```python
from build123d import *

# Parameters (mm, degrees)
SKETCH1_R           = 12.7
BOSS_EXTRUDE1_DEPTH = 12.7
SKETCH2_R           = 1.6256
CUT_EXTRUDE1_DEPTH  = 9.525
SKETCH3_R           = 9.525
CUT_EXTRUDE2_DEPTH  = 2.54
BOSS_EXTRUDE2_START = -12.7
BOSS_EXTRUDE2_DEPTH = 12.7
SKETCH10_R          = 1.651
CUT_EXTRUDE4_DEPTH  = 12.7
SKETCH11_R          = 9.525
CUT_EXTRUDE5_DEPTH  = 5.18668
CUT_EXTRUDE6_DEPTH  = 12.7
FILLET1_R           = 3.175
SKETCH16_R          = 8.255
CUT_EXTRUDE8_DEPTH  = 3.175
SKETCH17_R          = 1.2192
CUT_EXTRUDE9_DEPTH  = 4.33832
SKETCH18_R          = 3.81
CUT_EXTRUDE10_DEPTH = 2.54


with BuildPart() as part:
    # Sketch1 → Boss-Extrude1 (new body)
    with BuildSketch(Plane(origin=(0, 0, 0), x_dir=(1, 0, 0), z_dir=(0, 1, 0))):
        with Locations(Location((0, 0, 0), (0, 0, 270))):
            Circle(SKETCH1_R)
    extrude(amount=BOSS_EXTRUDE1_DEPTH)

    # Sketch2 → Cut-Extrude1 (cut)
    with BuildSketch(Plane.XZ):
        with Locations(Location((0, 0, 0), (0, 0, 270))):
            Circle(SKETCH2_R)
    extrude(amount=-CUT_EXTRUDE1_DEPTH, mode=Mode.SUBTRACT)

    # Sketch3 → Cut-Extrude2 (cut)
    with BuildSketch(Plane.XZ):
        with Locations(Location((0, 0, 0), (0, 0, 270))):
            Circle(SKETCH3_R)
    extrude(amount=-CUT_EXTRUDE2_DEPTH, mode=Mode.SUBTRACT)

    # Sketch5 → #2-56 Tapped Hole1 (revolve, cut)
    with BuildSketch(Plane(origin=(0, 3.81, 0), x_dir=(0, 1, 0), z_dir=(1, 0, 0))):
        Polygon((0, 0), (0, 13.74216509), (0.889, 13.208), (0.889, 0), align=None)
    revolve(axis=Axis((0, 3.81, -6.35), (0, 0, 1)), mode=Mode.SUBTRACT)

    # Sketch7 → Boss-Extrude2 (add)
    with BuildSketch(Plane(origin=(0, 12.7, 0), x_dir=(1, 0, 0), z_dir=(0, 1, 0)).offset(BOSS_EXTRUDE2_START)):
        with BuildLine():
            Line((-12.7, 152.4), (-12.7, 0))
            ThreePointArc((-12.7, 0), (0, 12.7), (12.7, 0))
            Line((12.7, 0), (12.7, 152.4))
            ThreePointArc((12.7, 152.4), (0, 165.1), (-12.7, 152.4))
        make_face()
    extrude(amount=BOSS_EXTRUDE2_DEPTH)

    # Sketch10 → Cut-Extrude4 (cut)
    with BuildSketch(Plane.XZ):
        with Locations(Location((0, -152.4, 0), (0, 0, 270))):
            Circle(SKETCH10_R)
    extrude(amount=-CUT_EXTRUDE4_DEPTH, mode=Mode.SUBTRACT)

    # Sketch11 → Cut-Extrude5 (cut)
    with BuildSketch(Plane.XZ):
        with Locations(Location((0, -152.4, 0), (0, 0, 270))):
            Circle(SKETCH11_R)
    extrude(amount=-CUT_EXTRUDE5_DEPTH, mode=Mode.SUBTRACT)

    # Sketch15 → Cut-Extrude6 (cut)
    with BuildSketch(Plane.XZ):
        with BuildLine():
            Line((-9.525, -35.469743879), (9.525, -16.419743879))
            Line((9.525, -16.419743879), (9.525, -8.400260413))
            ThreePointArc((9.525, -8.400260413), (0, -12.7), (-9.525, -8.400260413))
            Line((-9.525, -8.400260413), (-9.525, -35.469743879))
        make_face()
        Polygon((-9.525, -46.309871939), (9.525, -65.359871939), (9.525, -20.909871939), (-9.525, -39.959871939), align=None)
        Polygon((-9.525, -76.2), (9.525, -76.2), (9.525, -69.85), (-9.525, -50.8), align=None)
        Polygon((9.525, -82.55), (9.525, -76.2), (-9.525, -76.2), (-9.525, -101.6), align=None)
        Polygon((9.525, -131.490128061), (9.525, -87.040128061), (-9.525, -106.090128061), (-9.525, -112.440128061), align=None)
        with BuildLine():
            Line((9.525, -143.999739587), (9.525, -135.980256121))
            Line((9.525, -135.980256121), (-9.525, -116.930256121))
            Line((-9.525, -116.930256121), (-9.525, -143.999739587))
            ThreePointArc((-9.525, -143.999739587), (0, -139.7), (9.525, -143.999739587))
        make_face()
    extrude(amount=-CUT_EXTRUDE6_DEPTH, mode=Mode.SUBTRACT)

    # Fillet1
    fillet1_edges = [part.edges().sort_by_distance(p)[0] for p in [
        (9.525, 6.35, -143.999739587),
        (-9.525, 6.35, -143.999739587),
        (-9.525, 6.35, -116.930256121),
        (-9.525, 6.35, -35.469743879),
        (9.525, 6.35, -16.419743879),
        (9.525, 6.35, -8.400260413),
        (-9.525, 6.35, -8.400260413),
        (-9.525, 6.35, -46.309871939),
        (9.525, 6.35, -65.359871939),
        (9.525, 6.35, -20.909871939),
        (-9.525, 6.35, -101.6),
        (-9.525, 6.35, -50.8),
        (9.525, 6.35, -82.55),
        (9.525, 6.35, -131.490128061),
        (9.525, 6.35, -87.040128061),
        (-9.525, 6.35, -106.090128061),
        (-9.525, 6.35, -112.440128061),
    ]]
    fillet(fillet1_edges, radius=FILLET1_R)

    # Sketch16 → Cut-Extrude8 (cut)
    with BuildSketch(Plane.XZ.offset(-5.18668)):
        with Locations(Location((0, -152.4, 0), (0, 0, 270))):
            Circle(SKETCH16_R)
    extrude(amount=-CUT_EXTRUDE8_DEPTH, mode=Mode.SUBTRACT)

    # Sketch17 → Cut-Extrude9 (cut)
    with BuildSketch(Plane.XZ.offset(-8.36168)):
        with Locations(Location((-5.4599967, -152.4, 0), (0, 0, 270))):
            Circle(SKETCH17_R)
        with Locations(Location((5.4599967, -152.4, 0), (0, 0, 270))):
            Circle(SKETCH17_R)
    extrude(amount=-CUT_EXTRUDE9_DEPTH, mode=Mode.SUBTRACT)

    # Sketch18 → Cut-Extrude10 (cut)
    with BuildSketch(Plane.XZ.offset(-8.36168)):
        with Locations(Location((0, -152.4, 0), (0, 0, 270))):
            Circle(SKETCH18_R)
    extrude(amount=-CUT_EXTRUDE10_DEPTH, mode=Mode.SUBTRACT)


solid = part.part
```
Check sheet for the modelled part. Datum: model origin and axes. Units: mm. A direction names the side the tool comes from. Round coordinates to 2 decimals unless told otherwise and drop trailing zeros. Loops run counter-clockwise (first coordinate to the right, second up) from the corner with the lowest first, then second, coordinate; pieces in that order, holes last. Notation, with made-up numbers: M 20,-4.5 L 62,-4.5 A15 ccw 62,11.5 Z; hole C 69,-36 d4. An arc over 180 degrees is marked long. Answer as a JSON object with one key per item and string values.
1. Access from +Z, -Z, +X, -X, +Y, -Y to the whole of each face (thin tool, end or side, straight path). Record for faces 4 (the cylindrical face through (8.1, 6.4, -11.9)), 5 (the cylindrical face through (-0.279, 6.261, 12.697)), 6 (the flat face through (4, 5.187, -145)).
Reply:
{"face 4": "+Y, -Y", "face 5": "+Z, +Y, -Y", "face 6": "-Y"}
2. Scan lines: line 1 (X direction, y = 9.95, z = -152.4); line 2 (X direction, y = 4.5, z = -78) (3 decimals); line 3 (Z direction, x = -7.5, y = 9.5). Record each from-to range of solid material in increasing order.
Reply:
{"line 1": "x = -12.7 to -6.68, -4.24 to -3.81, 3.81 to 4.24, 6.68 to 12.7", "line 2": "x = -12.7 to -9.525, 9.525 to 12.7", "line 3": "z = -162.65 to -140.81, -121.64 to -114.47, -104.07 to -96.89, -55.51 to -48.33, -37.93 to -30.76, -11.59 to 10.25"}
3. Section check A-A (z = -129.5). Record the boundary of the cut face in (x, y) (3 decimals).
Reply:
{"outline": "M -12.7,0 L -9.525,0 L -9.525,12.7 L -12.7,12.7 Z; M 3.045,0 L 12.7,0 L 12.7,12.7 L 3.045,12.7 Z"}
4. Mould release check, pull along Z, two halves, no side actions. Record for faces 1 (the flat face through (12.7, 6, -75)), 2 (the flat face through (0, 2.54, -2)), 3 (the cylindrical face through (0.279, 6.261, -165.097)): pulls with the +Z half, pulls with the -Z half, needs draft (parallel to the pull), parting line crosses it, or undercut.
Reply:
{"face 1": "needs draft", "face 2": "undercut", "face 3": "pulls with the -Z half"}
5. Gauge pin test, flat ends, axial feed: P1, Ø1.5, axis at x = -5, y = 6, coming from the -Z side; P2, Ø2, axis at x = 5.46, z = -152.4, coming from the -Y side; P3, Ø1, axis at x = -0.5, z = 0.5, coming from the -Y side (3 decimals); P4, Ø5, axis at x = 4, y = 5, coming from the +Z side. Record the tip position at first contact, or that the pin passes through.
Reply:
{"P1": "stops at z = -164.37", "P2": "passes through", "P3": "stops at y = 9.525", "P4": "stops at z = 12.61"}
